CAD build for the part. Positions are in the model's coordinates, mm. Face numbers are marked on the shaded views. Give positions to 0.01 mm unless a question says otherwise; leave off trailing zeros. Write each loop counter-clockwise with the first axis right and the second up, starting at its lowest first coordinate (ties: lowest second). Pieces come first, ordered by that corner, then holes. Notation, with made-up numbers: (21, 36.5) - (30, 36.5) arc R23 cw to (30, 55.5) - close; hole circle Ø5 at (-4, 24). An arc over 180 degrees is marked (long way). Answer as a JSON object with one key per item and string values.
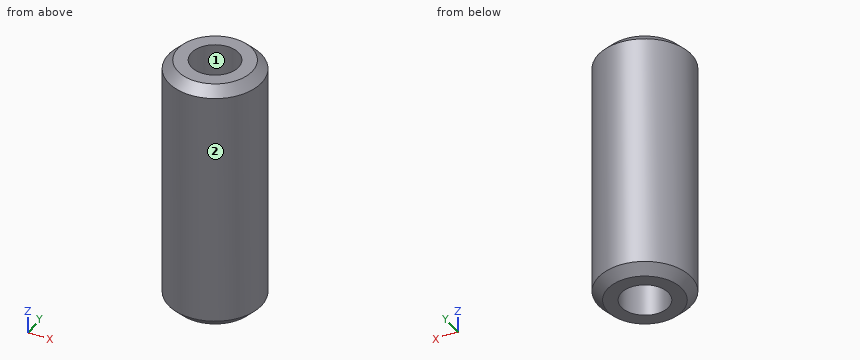
from build123d import *

# Parameters (mm, degrees)
SKETCH1_R           = 12.7
BOSS_EXTRUDE1_DEPTH = 69.85
SKETCH2_R           = 6.45
CUT_EXTRUDE1_DEPTH  = 73.122135992
CHAMFER1_SIZE       = 2.54


with BuildPart() as part:
    # Sketch1 → Boss-Extrude1 (new body)
    with BuildSketch(Plane.XY):
        Circle(SKETCH1_R)
    extrude(amount=BOSS_EXTRUDE1_DEPTH)

    # Sketch2 → Cut-Extrude1 (cut, through all)
    with BuildSketch(Plane(origin=(0, 0, 0), x_dir=(-1, 0, 0), z_dir=(0, 0, -1))):
        Circle(SKETCH2_R)
    extrude(amount=-CUT_EXTRUDE1_DEPTH, mode=Mode.SUBTRACT)

    # Chamfer1
    chamfer1_edges = [part.edges().sort_by_distance(p)[0] for p in [
        (-12.7, 0, 0),
        (-12.7, 0, 69.85),
    ]]
    chamfer(chamfer1_edges, length=CHAMFER1_SIZE)


solid = part.part
Item 1: Mould opens along Y. For the marked faces 1 and 2 say: +Y half, -Y half, draft (parallel to the pull), parting line (faces both ways), or undercut.
Entries:
{"face 1": "undercut", "face 2": "parting line"}
Item 2: Flat gauge pins, fed straight in: P1, Ø8, axis at x = -10, z = 58, coming from the -Y side; P2, Ø2, axis at y = -8.5, z = 10.5, coming from the -X side; P3, Ø6, axis at y = -3.5, z = 58, coming from the +X side. Where does each tip first touch, or does it go through?
Entries:
{"P1": "y = -11.19", "P2": "x = -10.25", "P3": "x = 12.69"}
Item 3: Cut at C-C (z = 23.5). Give the cut face in (x, y), and give its area (3 significant figures).
Entries:
{"outline": "circle Ø25.4 at (0, 0); hole circle Ø12.9 at (0, 0)", "area": "376 mm2"}
Item 4: Probe line 1 (Y direction, x = 0, z = 47); line 2 (X direction, y = 2.5, z = 42); line 3 (Y direction, x = 4.25, z = 34.5). List the from-to ranges inside material, lowest first. Write a range as from..to.
Entries:
{"line 1": "-12.7..-6.45, 6.45..12.7", "line 2": "-12.45..-5.95, 5.95..12.45", "line 3": "-11.97..-4.85, 4.85..11.97"}
Item 5: Cut at A-A (x = 0). Give the cut face in (y, z), and give its area (3 significant figures).
Entries:
{"outline": "(-12.7, 2.54) - (-10.16, 0) - (-6.45, 0) - (-6.45, 69.85) - (-10.16, 69.85) - (-12.7, 67.31) - close; (6.45, 0) - (10.16, 0) - (12.7, 2.54) - (12.7, 67.31) - (10.16, 69.85) - (6.45, 69.85) - close", "area": "860 mm2"}
